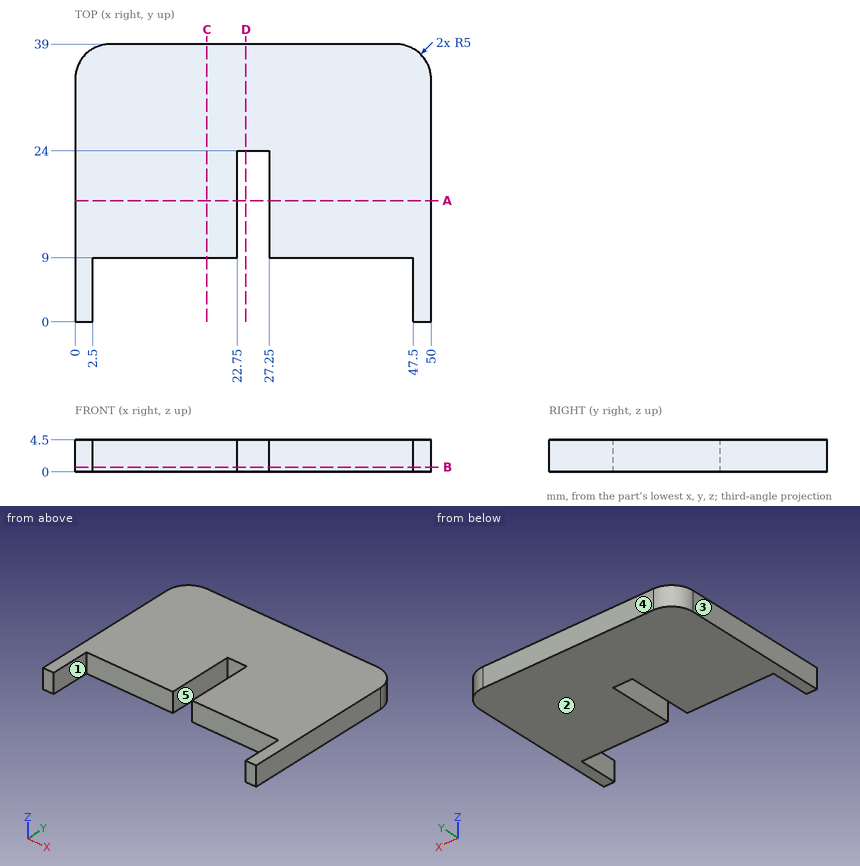
Geometry: see drawing. Coordinates: mm, zero at the bounding-box minimum. A direction names the side the tool comes from. Give positions to 0.01 mm unless a question says otherwise; leave off trailing zeros. Loops run counter-clockwise (first coordinate to the right, second up) from the corner with the lowest first, then second, coordinate; pieces in that order, holes last. Notation, with made-up numbers: (-9, 23) -> (7, 23) arc R22 cw to (7, 61) -> close; hole circle Ø10 at (52.5, 5). An arc over 180 degrees is marked (long way). Answer as a JSON object with one key per item and string values. Group by question number.
Item 1: Line query: probe 1 along X at (y, z) = (16, 1.95); probe 2 along X at (y, z) = (6.5, 0.6); probe 3 along Y at (x, z) = (28, 2.6). Output: solid intervals per line, ascending.
Item 2: Cut plane A-A, the plane y = 17. Return the cut outline in (x, z).
Item 3: Reachability of the marked faces 4 and 5 from +Z, -Z, +X, -X, +Y, -Y: full face, straight path, thin tool, end or side. Return the list, or none.
Item 4: Cut plane D-D, the plane x = 24. Return the cut outline in (y, z), and give its area (3 significant figures).
Item 5: Cut plane C-C, the plane x = 18.5. Return the cut outline in (y, z), and give its area (3 significant figures).
Item 6: Cut plane B-B, the plane z = 0.65. Return the cut outline in (x, y).
Item 7: Pin query (flat end, axial travel): P1, Ø1.3, axis at x = 39.5, z = 1.5, coming from the -Y side. Return the tip coordinate at first contact, or that it passes through.
Item 8: Pull-direction query (X, two-part tool) for the marked faces 1, 2 and 3; classes: released by +X, released by -X, zero draft, split by the parting line, or undercut.
Checks:
{
 "1": {"probe 1": "x = 0 to 22.75, 27.25 to 50", "probe 2": "x = 0 to 2.5, 47.5 to 50", "probe 3": "y = 9 to 39"},
 "2": {"outline": "(0, 0) -> (22.75, 0) -> (22.75, 4.5) -> (0, 4.5) -> close; (27.25, 0) -> (50, 0) -> (50, 4.5) -> (27.25, 4.5) -> close"},
 "3": {"face 4": "+Z, -Z, +X, -X, +Y", "face 5": "+Z, -Z, -Y"},
 "4": {"outline": "(24, 0) -> (39, 0) -> (39, 4.5) -> (24, 4.5) -> close", "area": "67.5 mm²"},
 "5": {"outline": "(9, 0) -> (39, 0) -> (39, 4.5) -> (9, 4.5) -> close", "area": "135 mm²"},
 "6": {"outline": "(0, 0) -> (2.5, 0) -> (2.5, 9) -> (22.75, 9) -> (22.75, 24) -> (27.25, 24) -> (27.25, 9) -> (47.5, 9) -> (47.5, 0) -> (50, 0) -> (50, 34) arc R5 ccw to (45, 39) -> (5, 39) arc R5 ccw to (0, 34) -> close"},
 "7": {"P1": "stops at y = 9"},
 "8": {"face 1": "undercut", "face 2": "zero draft", "face 3": "released by -X"}
}
